Could you check a few things on this drawing? It's one solid part, dimensions in mm from its lowest x, y, z. Round coordinates to 2 decimals unless told otherwise and drop trailing zeros. Write each loop counter-clockwise with the first axis right and the second up, starting at its lowest first coordinate (ties: lowest second). Pieces come first, ordered by that corner, then holes. Notation, with made-up numbers: (-30.75, 51.25) - (2.25, 51.25) arc R19 ccw to (2.25, 84.25) - close; hole circle Ø1 at (80.25, 10.25). An arc over 180 degrees is marked (long way). Use one line per item in the form item = value. Start each with the question number.
1. Will this pin go through, and if not, where does the flat tip stop? pin 1 (5.5 mm diameter, centred on x = 5, z = 5, fed in from -Y).
2. If I drill on line 1 along X through (y, z) = (0.7, 49.2); line 2 along Z through (x, y) = (107, 1.4); line 3 along X through (y, z) = (0.2, 6), over which ranges is the centre line in solid material (lowest first)?
3. I want a section at B-B, the plane x = 5. List the corners of the cut face in (y, z) for me.
4. I want a section at A-A, the plane z = 49.2. List the corners of the cut face in (x, y) for me, plus the area to 3 significant figures.
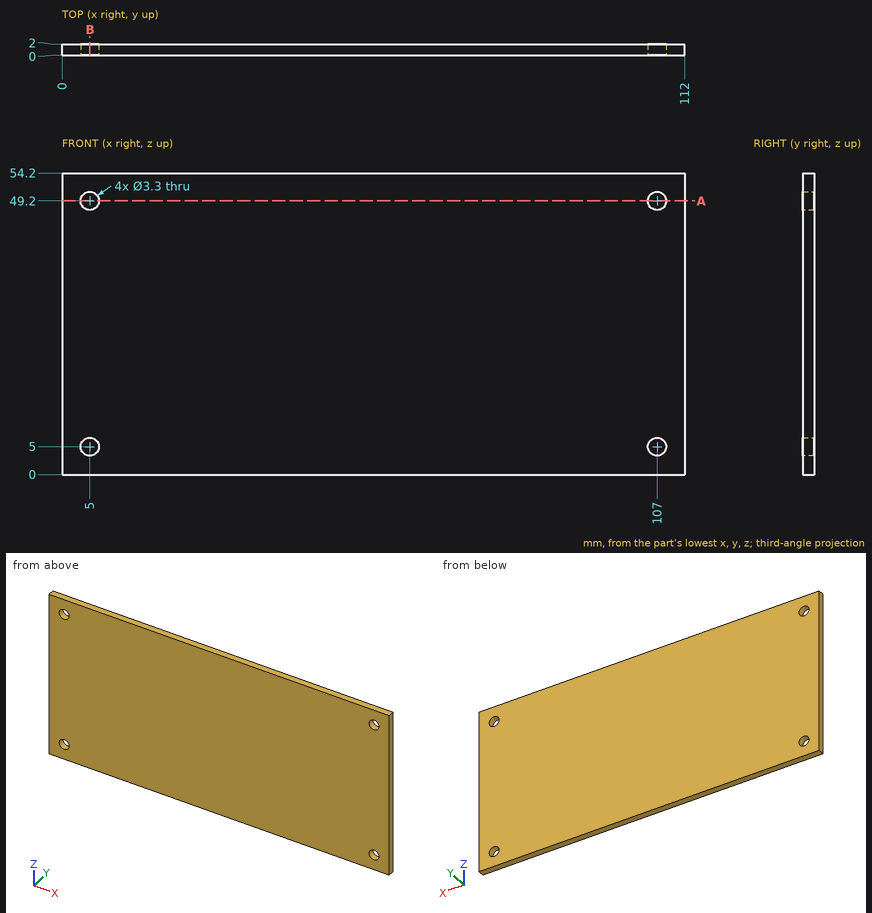
Model answer:
q1.pin_1 = 0
q2.line_1 = 0 to 3.35, 6.65 to 105.35, 108.65 to 112
q2.line_2 = 0 to 3.35, 6.65 to 47.55, 50.85 to 54.2
q2.line_3 = 0 to 3.69, 6.31 to 105.69, 108.31 to 112
q3.outline = (0, 0) - (2, 0) - (2, 3.35) - (0, 3.35) - close; (0, 6.65) - (2, 6.65) - (2, 47.55) - (0, 47.55) - close; (0, 50.85) - (2, 50.85) - (2, 54.2) - (0, 54.2) - close
q4.outline = (0, 0) - (3.35, 0) - (3.35, 2) - (0, 2) - close; (6.65, 0) - (105.35, 0) - (105.35, 2) - (6.65, 2) - close; (108.65, 0) - (112, 0) - (112, 2) - (108.65, 2) - close
q4.area = 211 mm2
